Can you work these out from the model? Positions are in its coordinate system, mm. A direction names the side the tool comes from. Round coordinates to 2 decimals unless told otherwise and drop trailing zeros. Loops run counter-clockwise (first coordinate to the right, second up) from the corner with the lowest first, then second, coordinate; pieces in that order, holes last. Notation, with made-up numbers: M -33.5,57.25 L 23.5,57.25 A19 ccw 23.5,75.25 Z; hole C 80.25,63 d4. An arc over 180 degrees is marked long. Return JSON: item names as keys, results as strings.
Autodesk Inventor part; units mm, degrees
ref_plane "YZ Plane" through (0, 0, 0) normal (1, 0, 0) x (0, 1, 0)
ref_plane "XZ Plane" through (0, 0, 0) normal (0, 1, 0) x (-1, 0, 0)
ref_plane "XY Plane" through (0, 0, 0) normal (0, 0, 1) x (1, 0, 0)
sketch "Sketch1" plane through (0, 0, 0) normal (0, 0, 1) x (1, 0, 0)
  line L0 (0, 0) -> (146.881681, 0)
  line L1 (146.881681, -25.4) -> (0, -25.4)
  line L2 (0, 0) -> (73.44084, 0)
  line L3 (73.44084, 0) -> (73.44084, -3.175)
  line L4 (73.44084, -3.175) -> (71.84064, -3.175)
  line L5 (71.84064, -3.175) -> (71.84064, -9.525)
  line L6 (71.84064, -9.525) -> (75.01564, -9.525)
  line L7 (75.01564, -9.525) -> (75.01564, -3.175)
  line L8 (75.01564, -3.175) -> (73.44084, -3.175)
  line L9 (73.44084, -25.4) -> (73.44084, -22.225)
  line L10 (73.44084, -22.225) -> (71.84064, -22.225)
  line L11 (71.84064, -22.225) -> (71.84064, -15.875)
  line L12 (71.84064, -15.875) -> (75.01564, -15.875)
  line L13 (75.01564, -15.875) -> (75.01564, -22.225)
  line L14 (75.01564, -22.225) -> (73.44084, -22.225)
  dimension "d8" = 6.7564
sketch "Sketch3" plane through (0, 3.175, 76.2) normal (0, 1, 0) x (1, 0, 0)
  line L0 (0, 0) -> (25.4, 0)
  circle A0 centre (12.7, 44.45) radius 3.3782
  circle A1 centre (12.7, 22.225) radius 3.3782
  line L1 (0, 76.2) -> (0, 73.025)
  dimension "d21" = 6.7564
  dimension "d22" = 6.7564
  dimension "d23" = 12.7
  dimension "d24" = 22.225
  dimension "d25" = 22.225
sketch "Sketch1 outline for Plate1" plane through (0, 0, 0) normal (0, 0, 1) x (1, 0, 0)
  line L0 (0, 0) -> (0, 76.2)
  line L1 (25.4, 0) -> (0, 0)
  line L2 (0, 76.2) -> (25.4, 76.2)
  line L3 (25.4, 76.2) -> (25.4, 0)
  circle A0 centre (12.7, 22.225) radius 3.3782
  circle A1 centre (12.7, 44.45) radius 3.3782
extrude "Plate1" add sketch "Sketch1 outline for Plate1" along normal blind 3.175
sketch "Sketch2" plane through (25.4, 3.175, 0) normal (0, -1, 0) x (1, 0, 0)
  line L0 (-25.4, 0) -> (0, 0)
  line L1 (0, 0) -> (0, 76.2)
  line L2 (0, 76.2) -> (-25.4, 76.2)
  line L3 (-25.4, 76.2) -> (-25.4, 0)
edge flange "Flange1" height 76.2 angle 90 thickness 3.175 bend radius 3.175 thickness toward (0, -1, 0) relief tear relief width 3.175 relief depth 1.5875 edges at (12.7, 0, 3.175) wall of the first edge with corners at (0, 3.175, 0) (25.4, 3.175, 0) (25.4, 3.175, 76.2) (0, 3.175, 76.2)
bend "Bend1"
corner "Corner1"
extrude "Cut1" cut sketch "Sketch3" against normal blind 3.175
equation "\"d11\" = BendReliefWidth"
equation "\"d12\" = BendReliefDepth"
equation "\"d13\" = MinimumRemnant"
equation "\"d14\" = BendRadius"
equation "\"d17\" = BendRadius"
equation "\"d18\" = CornerReliefSize"
equation "\"d19\" = GapSize"
equation "\"d20\" = JacobiRadiusSize"
equation "\"BendRadius\" = Thickness"
equation "\"BendReliefWidth\" = Thickness"
equation "\"BendReliefDepth\" = 0.5 * Thickness"
equation "\"CornerReliefSize\" = 4 * Thickness"
equation "\"MinimumRemnant\" = 2 * Thickness"
equation "\"TransitionRadius\" = BendRadius"
equation "\"JacobiRadiusSize\" = BendRadius"
equation "\"GapSize\" = Thickness"
equation "\"d10\" = BendRadius"
equation "\"d6\" = Thickness"
properties part number "Gusset 4" material "Aluminum 6061"
Q1. If I drill on line 1 along Y through (x, z) = (12.7, 1.05); line 2 along X through (y, z) = (1.3, 31.75); line 3 along Y through (x, z) = (12.7, 1.45), over which ranges is the centre line in solid material (lowest first)?
Results:
{"line 1": "y = 2.85 to 18.85, 25.6 to 41.07, 47.83 to 76.2", "line 2": "x = 0 to 9.32, 16.08 to 25.4", "line 3": "y = 2.31 to 18.85, 25.6 to 41.07, 47.83 to 76.2"}
Q2. Suppose I cut it at D-D, the plane x = 8.25. Please give me the cut outline in (y, z) (3 decimals).
Results:
{"outline": "M 0,6.35 A6.35 ccw 6.35,0 L 76.2,0 L 76.2,3.175 L 6.35,3.175 A3.175 cw 3.175,6.35 L 3.175,76.2 L 0,76.2 Z"}
Q3. Thinking about a two-plate mould opening in X: for faces 1 (the cylindrical face through (12.26, 41.1, 1.57)), 2 (the flat face through (25.4, 1, 21)), 3 (the flat face through (15.3, 41.8, 0)), 4 (the flat face through (0, 1, 21)), which applies, pulls with the +X half, pulls with the -X half, needs draft (parallel to the pull), parting line crosses it, or undercut?
Results:
{"face 1": "undercut", "face 2": "pulls with the +X half", "face 3": "needs draft", "face 4": "pulls with the -X half"}
Q4. Suppose I cut it at A-A, the plane x = 12.7. Please give me the cut outline in (y, z) (3 decimals).
Results:
{"outline": "M 0,6.35 A6.35 ccw 6.35,0 L 18.847,0 L 18.847,3.175 L 6.35,3.175 A3.175 cw 3.175,6.35 L 3.175,28.372 L 0,28.372 Z; M 0,35.128 L 3.175,35.128 L 3.175,50.597 L 0,50.597 Z; M 0,57.353 L 3.175,57.353 L 3.175,76.2 L 0,76.2 Z; M 25.603,0 L 41.072,0 L 41.072,3.175 L 25.603,3.175 Z; M 47.828,0 L 76.2,0 L 76.2,3.175 L 47.828,3.175 Z"}
Q5. Suppose I cut it at B-B, the plane y = 44.45. Please give me the cut outline in (x, z) (3 decimals), plus the area to 3 significant figures.
Results:
{"outline": "M 0,0 L 9.322,0 L 9.322,3.175 L 0,3.175 Z; M 16.078,0 L 25.4,0 L 25.4,3.175 L 16.078,3.175 Z", "area": "59.2 mm2"}
Q6. I'm going to push flat-ended pins straight in: pin 1 Ø12.5 at (x, z) = (15.5, 54.5) entering from +Y (3 decimals); pin 2 Ø5 at (x, y) = (3.5, 37) entering from +Z (3 decimals). Where does each tip first touch, or does it pass through?
Results:
{"pin 1": "stops at y = 3.175", "pin 2": "stops at z = 3.175"}
Q7. On a 3-axis mill with a long thin cutter (end or side, diameter ignored), from which of +Z, -Z, +X, -X, +Y, -Y can I reach the whole of each face in a straight line? I mean faces 5 (the cylindrical face through (12.26, 1.61, 50.626)), 6 (the flat face through (15.3, 41.8, 3.175)). Say none if no direction works.
Results:
{"face 5": "+Y, -Y", "face 6": "+Z, +X, -X, +Y"}
